Part model, mm, in its own coordinate system. Face numbers are marked on the shaded views. Round coordinates to 2 decimals unless told otherwise and drop trailing zeros. Write each loop counter-clockwise with the first axis right and the second up, starting at its lowest first coordinate (ties: lowest second). Pieces come first, ordered by that corner, then holes.
```python
from build123d import *

# Parameters (mm, degrees)
SKETCH1_W           = 45
SKETCH1_H           = 45
BOSS_EXTRUDE1_DEPTH = 1.6
SKETCH2_W           = 40
SKETCH2_H           = 34
BOSS_EXTRUDE2_DEPTH = 3.5
SKETCH4_W           = 20.66
SKETCH4_H           = 2.5
BOSS_EXTRUDE3_DEPTH = 2.8
SKETCH5_W           = 0.7
SKETCH5_H           = 0.7
BOSS_EXTRUDE4_DEPTH = 5.95
CUT_EXTRUDE1_DEPTH  = 0.1


with BuildPart() as part:
    # Sketch1 → Boss-Extrude1 (new body)
    with BuildSketch(Plane(origin=(0, 0, 0), x_dir=(1, 0, 0), z_dir=(0, 1, 0))):
        Rectangle(SKETCH1_W, SKETCH1_H)
    extrude(amount=BOSS_EXTRUDE1_DEPTH)

    # Sketch2 → Boss-Extrude2 (add)
    with BuildSketch(Plane(origin=(0, 1.6, 0), x_dir=(1, 0, 0), z_dir=(0, 1, 0))):
        Rectangle(SKETCH2_W, SKETCH2_H)
    extrude(amount=BOSS_EXTRUDE2_DEPTH)

    # Sketch4 → Boss-Extrude3 (add)
    with BuildSketch(Plane.XZ):
        with Locations((0, 19.825)):
            Rectangle(SKETCH4_W, SKETCH4_H)
    boss_extrude3 = extrude(amount=BOSS_EXTRUDE3_DEPTH)

    # Sketch5 → Boss-Extrude4 (add)
    with BuildSketch(Plane.XZ.offset(2.8)):
        with Locations((-8.89, 19.825)):
            Rectangle(SKETCH5_W, SKETCH5_H)
        with Locations((-6.35, 19.825)):
            Rectangle(SKETCH5_W, SKETCH5_H)
        with Locations((-3.81, 19.825)):
            Rectangle(SKETCH5_W, SKETCH5_H)
        with Locations((-1.27, 19.825)):
            Rectangle(SKETCH5_W, SKETCH5_H)
        with Locations((1.27, 19.825)):
            Rectangle(SKETCH5_W, SKETCH5_H)
        with Locations((3.81, 19.825)):
            Rectangle(SKETCH5_W, SKETCH5_H)
        with Locations((6.35, 19.825)):
            Rectangle(SKETCH5_W, SKETCH5_H)
        with Locations((8.89, 19.825)):
            Rectangle(SKETCH5_W, SKETCH5_H)
    boss_extrude4 = extrude(amount=BOSS_EXTRUDE4_DEPTH)

    # Sketch6 → Cut-Extrude1 (cut)
    with BuildSketch(Plane(origin=(0, 5.1, 0), x_dir=(1, 0, 0), z_dir=(0, 1, 0))):
        with BuildLine():
            Line((-15.85, 15.65), (15.85, 15.65))
            ThreePointArc((15.85, 15.65), (17.617766953, 14.917766953), (18.35, 13.15))
            Line((18.35, 13.15), (18.35, -8.25))
            ThreePointArc((18.35, -8.25), (17.617766953, -10.017766953), (15.85, -10.75))
            Line((15.85, -10.75), (-15.85, -10.75))
            ThreePointArc((-15.85, -10.75), (-17.617766953, -10.017766953), (-18.35, -8.25))
            Line((-18.35, -8.25), (-18.35, 13.15))
            ThreePointArc((-18.35, 13.15), (-17.617766953, 14.917766953), (-15.85, 15.65))
        make_face()
    extrude(amount=-CUT_EXTRUDE1_DEPTH, mode=Mode.SUBTRACT)

    # Mirror1: Boss-Extrude3, Boss-Extrude4 across plane
    add(boss_extrude3.mirror(Plane.XY))
    add(boss_extrude4.mirror(Plane.XY))


solid = part.part
```
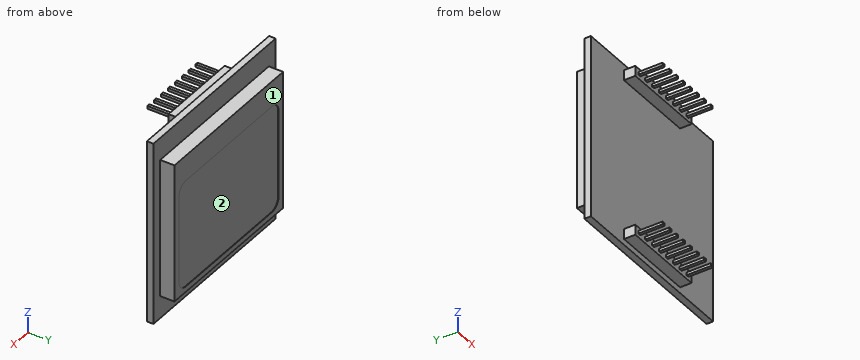
Q1. Cut at D-D on x = -12.5. Write the cut outline in (y, z), plus the area to 3 significant figures.
Values follow:
outline: (0, -22.5) - (1.6, -22.5) - (1.6, -17) - (5.1, -17) - (5.1, -15.65) - (5, -15.65) - (5, 10.75) - (5.1, 10.75) - (5.1, 17) - (1.6, 17) - (1.6, 22.5) - (0, 22.5) - close
area: 188 mm2
Q2. Cut at A-A on y = -1. Write the cut outline in (x, z) (3 decimals), plus the area to 3 significant figures.
Values follow:
outline: (-10.33, -21.075) - (10.33, -21.075) - (10.33, -18.575) - (-10.33, -18.575) - close; (-10.33, 18.575) - (10.33, 18.575) - (10.33, 21.075) - (-10.33, 21.075) - close
area: 103 mm2
Q3. Mould opens along Z. For the marked faces 1 and 2 say: +Z half, -Z half, draft (parallel to the pull), parting line (faces both ways), or undercut.
Values follow:
face 1: draft
face 2: undercut
Q4. Cut at C-C on z = 15.5. Write the cut outline in (x, y).
Values follow:
outline: (-22.5, 0) - (22.5, 0) - (22.5, 1.6) - (20, 1.6) - (20, 5.1) - (-20, 5.1) - (-20, 1.6) - (-22.5, 1.6) - close
Q5. Cut at B-B on x = 19. Write the cut outline in (y, z).
Values follow:
outline: (0, -22.5) - (1.6, -22.5) - (1.6, -17) - (5.1, -17) - (5.1, 17) - (1.6, 17) - (1.6, 22.5) - (0, 22.5) - close
Q6. Drop flat-ended pins along their axis: pin 1 (6 mm diameter, centred on x = 14, z = 5.5, fed in from -Y); pin 2 (4 mm diameter, centred on x = -14.5, z = 8.5, fed in from +Y); pin 3 (1.7 mm diameter, centred on y = 3, z = 4, fed in from -X). Give the stop position or say it passes through.
Values follow:
pin 1: stops at y = 0
pin 2: stops at y = 5
pin 3: stops at x = -20
Q7. Wall check: L1, parallel to Z at x = 4, y = -7 (3 decimals); L2, parallel to Z at x = 4, y = -2.75 (3 decimals); L3, parallel to Z at x = -19, y = 2. Give the ranges that are in metal, low to high.
Values follow:
L1: z = -20.175 to -19.475, 19.475 to 20.175
L2: z = -21.075 to -18.575, 18.575 to 21.075
L3: z = -17 to 17
